```python
from build123d import *

# Parameters (mm, degrees)
BOSS_EXTRUDE1_DEPTH = 2


with BuildPart() as part:
    # Sketch1 → Boss-Extrude1 (new body)
    with BuildSketch(Plane.XY):
        with BuildLine():
            Line((-24.999999472, 3), (-12, 3))
            ThreePointArc((-12, 3), (-11.292893219, 2.707106781), (-11, 2))
            Line((-11, 2), (-11, 1))
            Line((-11, 1), (-17, 1))
            Line((-17, 1), (-17, -1))
            Line((-17, -1), (-11, -1))
            Line((-11, -1), (-11, -2))
            ThreePointArc((-11, -2), (-11.292893219, -2.707106781), (-12, -3))
            Line((-12, -3), (-24.999999472, -3))
            Line((-24.999999472, -3), (-24.999999472, -10))
            ThreePointArc((-24.999999472, -10), (-25.292892691, -10.707106781), (-25.999999472, -11))
            Line((-25.999999472, -11), (-28.982753492, -11))
            ThreePointArc((-28.982753492, -11), (-31, 0), (-28.982753492, 11))
            Line((-28.982753492, 11), (-25.999999472, 11))
            ThreePointArc((-25.999999472, 11), (-25.292892691, 10.707106781), (-24.999999472, 10))
            Line((-24.999999472, 10), (-24.999999472, 3))
        make_face()
    extrude(amount=BOSS_EXTRUDE1_DEPTH)


solid = part.part
```
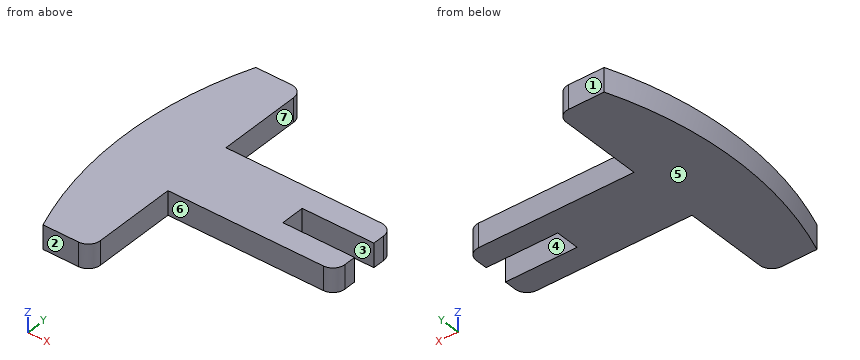
Model file for the job. Use its own axes, mm. Face numbers are marked on the shaded views. A direction names the side the tool comes from. Coordinates: 2 decimals unless noted, no trailing zeros. Order: outer loops, then holes, each group sorted by start corner. A loop starts at its lowest first (then second) coordinate and runs counter-clockwise, first axis right, second up. Notation, with made-up numbers: (-12, 78) -> (31, 78) arc R10 cw to (31, 96) -> close; hole circle Ø2 at (34.5, 22.5). An arc over 180 degrees is marked (long way). Return JSON: item names as keys, results as strings.
Item 1: Slice it at A-A (x = -16.5). Write the cut outline in (y, z), then the cut area to 3 significant figures.
Model answer:
{"outline": "(-3, 0) -> (-1, 0) -> (-1, 2) -> (-3, 2) -> close; (1, 0) -> (3, 0) -> (3, 2) -> (1, 2) -> close", "area": "8.00 mm²"}
Item 2: Slice it at B-B (z = 0.85). Write the cut outline in (x, y), then the cut area to 3 significant figures.
Model answer:
{"outline": "(-28.98, -11) -> (-26, -11) arc R1 ccw to (-25, -10) -> (-25, -3) -> (-12, -3) arc R1 ccw to (-11, -2) -> (-11, -1) -> (-17, -1) -> (-17, 1) -> (-11, 1) -> (-11, 2) arc R1 ccw to (-12, 3) -> (-25, 3) -> (-25, 10) arc R1 ccw to (-26, 11) -> (-28.98, 11) arc R31 ccw to start", "area": "189 mm²"}
Item 3: Slice it at C-C (y = 0). Write the cut outline in (x, z), then the cut area to 3 significant figures.
Model answer:
{"outline": "(-31, 0) -> (-17, 0) -> (-17, 2) -> (-31, 2) -> close", "area": "28.0 mm²"}
Item 4: 3-axis set-ups, long thin cutter, end or side, ignore diameter. For the marked faces 5, 6 and 7: which of +Z, -Z, +X, -X, +Y, -Y reach the whole face in a straight line?
Model answer:
{"face 5": "-Z, +X, -X, +Y, -Y", "face 6": "+Z, -Z, +X, -Y", "face 7": "+Z, -Z, +X, +Y"}
Item 5: Slice it at D-D (y = -3.5). Write the cut outline in (x, z).
Model answer:
{"outline": "(-30.8, 0) -> (-25, 0) -> (-25, 2) -> (-30.8, 2) -> close"}
Item 6: Pin check, flat tip, straight feed: P1, Ø1, axis at x = -20.5, z = 1, coming from the +Y side. Stop position of the tip, or through.
Model answer:
{"P1": "stops at y = 3"}
Item 7: Wall check: line 1 along Y through (x, z) = (-14, 0.25); line 2 along Y through (x, z) = (-21.5, 1.3); line 3 along X through (y, z) = (0.25, 0.5). Give the ranges that are in metal, low to high. Write a range as from..to.
Model answer:
{"line 1": "y = -3..-1, 1..3", "line 2": "y = -3..3", "line 3": "x = -31..-17"}
Item 8: Mould opens along Y. For the marked faces 1, 2, 3 and 4 say: pulls with the +Y half, pulls with the -Y half, needs draft (parallel to the pull), parting line crosses it, or undercut.
Model answer:
{"face 1": "pulls with the +Y half", "face 2": "pulls with the -Y half", "face 3": "undercut", "face 4": "undercut"}
